Autodesk Inventor part; units mm, degrees
ref_plane "YZ Plane" through (0, 0, 0) normal (1, 0, 0) x (0, 1, 0)
ref_plane "XZ Plane" through (0, 0, 0) normal (0, 1, 0) x (-1, 0, 0)
ref_plane "XY Plane" through (0, 0, 0) normal (0, 0, 1) x (1, 0, 0)
sketch "スケッチ1" plane through (0, 0, 0) normal (0, 1, 0) x (-1, 0, 0)
  circle A0 centre (0, 0) radius 34.996
  circle A1 centre (0, 18) radius 10
  line L0 (48.9944, 0) -> (-48.9944, 0)
  line L1 (-14, 8) -> (14, 8)
  line L2 (14, 8) -> (14, 32.0737)
  line L3 (14, 32.0737) -> (-14, 32.0737)
  line L4 (-14, 32.0737) -> (-14, 8)
  line L5 (-14, 8) -> (14, 32.0737) construction
  line L6 (14, 8) -> (-14, 32.0737) construction
  point P0 (10, 25)
  point P1 (-10, 25)
  point P2 (0, 20.0368)
  dimension "d0" = 25
  dimension "d1" = 10
  dimension "d2" = 10
  dimension "d3" = 69.992
  dimension "d5" = 20
  dimension "d7" = 18
  dimension "d8" = 4
extrude "押し出し1" add sketch "スケッチ1" along normal blind 27 contours L3 A0 | A1 | L2 L1 L4 L3
hole "穴1" at (-10, 0, 25) at (10, 0, 25) direction (0, 1, 0) diameter 3.4 end through all
sketch "スケッチ2" plane through (0, 0, 0) normal (0, -1, 0) x (1, 0, 0)
  circle A0 centre (3.5, 18) radius 7 construction
  circle A1 centre (-7, 18) radius 3.5 construction
  line L0 (-3.5, 18) -> (3.5, 18) construction
  line L1 (-3.5, 11) -> (3.5, 11)
  line L2 (3.5, 25) -> (-3.5, 25)
  arc A2 (-3.5, 25) -> (-3.5, 11) centre (-3.5, 18) ccw
  arc A3 (3.5, 11) -> (3.5, 25) centre (3.5, 18) ccw
  point P0 (0, 0)
  point P1 (0, 18)
  point P2 (-10.5, 18)
  dimension "d31" = 7
  dimension "d30" = 14
  dimension "d32" = 7
extrude "押し出し2" cut sketch "スケッチ2" against normal through all
sketch "スケッチ3" plane through (0, 0, 0) normal (0, -1, 0) x (1, 0, 0)
  line L0 (14, 8) -> (-14, 8)
  line L1 (14, -21) -> (-14, -21)
  line L2 (-14, -21) -> (-14, 21)
  line L3 (-14, 21) -> (14, 21)
  line L4 (14, 21) -> (14, -21)
  line L5 (14, -21) -> (-14, 21) construction
  line L6 (-14, -21) -> (14, 21) construction
  circle A0 centre (-10, 25) radius 1.7
  point P0 (0, 0)
  point P1 (-14, 8)
  dimension "d25" = 4
extrude "押し出し3" cut sketch "スケッチ3" against normal blind 15 contours L0 L2 L3 L4
fillet "フィレット2" radius 2 8 edges at (14, 21, 8) (14, 7.5, 21) (-14, 7.5, 21) (-14, 21, 8) (14, 13.5, 32.0737) (-14, 13.5, 32.0737) (9.8246, 7.5, 21) (-9.8246, 7.5, 21)
equation "\"d32\" = 0.5 * d30"
properties part number "scara-base13" material "ABS プラスチック"
Design review of the part built by this model. Coordinates are the model's own, in mm. A direction names the side the tool comes from. Give positions to 0.01 mm unless a question says otherwise; leave off trailing zeros. Write each loop counter-clockwise with the first axis right and the second up, starting at its lowest first coordinate (ties: lowest second). Pieces come first, ordered by that corner, then holes. Notation, with made-up numbers: (85, 1.25) - (93, 1.25) arc R17 cw to (93, 23.25) - close; hole circle Ø10 at (-6.75, -14.75). An arc over 180 degrees is marked (long way). Return JSON: item names as keys, results as strings. Group by question number.
(1) We need section B-B, the plane y = 2.5. Give the boundary of the cut face in (x, z), then the cut area to 3 significant figures.
(2) We need section C-C, the plane z = 23.75. Give the boundary of the cut face in (x, y).
(3) We need section D-D, the plane y = 17.5. Give the boundary of the cut face in (x, z), then the cut area to 3 significant figures.
(4) To check wall thickness, follow probe 1 along X at (y, z) = (11, 26); probe 2 along Z at (x, y) = (-1, 22.5); probe 3 along Z at (x, y) = (10, 13.5). State the ranges of each line that lie inside material, in increasing order.
(5) Mouldability with a two-part tool opening along X and no side actions: class faces 1 (the flat face through (0, 21, 8)), 2 (the cylindrical face through (13.43, 21.08, 8.6)), 3 (the cylindrical face through (0.182, 13.311, 34.996)), 4 (the flat face through (0, 13, 25)) as +X half, -X half, draft (parallel to the pull), parting line (faces both ways), or undercut.
(6) We need section A-A, the plane x = -10. Give the boundary of the cut face in (y, z).
(7) Insertion check: pin 1 (6 mm diameter, centred on x = 6.5, z = 20.5, fed in from +Y); pin 2 (2 mm diameter, centred on x = 3, y = 11, fed in from -Z); pin 3 (5.5 mm diameter, centred on x = 1.5, y = 21.5, fed in from +Z); pin 4 (1.1 mm diameter, centred on x = -11.5, y = 4, fed in from -Z). Each pin has a flat end and moves straight along its axis. Give the tip position at first contact, or say it passes through.
(8) Machinability: for faces 5 (the cylindrical face through (-13.4, 7.6, 21.57)), 6 (the cylindrical face through (10.03, 7.4, 21.24)), 7 (the cylindrical face through (10.13, 16.31, 20.25)), 8 (the cylindrical face through (13.43, 7.6, 21.6)), 9 (the flat face through (-11.5, 7.4, 21)), which of the approach directions +Z, -Z, +X, -X, +Y, -Y give a long, thin tool a straight path to every point of the face, cutting with its end or side? Answer none if there is none.
Reported:
{
 "1": {"outline": "(-14, 23) arc R2 ccw to (-12, 21) - (-10.98, 21) arc R2 ccw to (-9.32, 21.89) arc R7 cw to (-3.5, 25) - (3.5, 25) arc R7 cw to (9.32, 21.89) arc R2 ccw to (10.98, 21) - (12, 21) arc R2 ccw to (14, 23) - (14, 30.74) arc R2 ccw to (12.73, 32.6) arc R35 ccw to (-12.73, 32.6) arc R2 ccw to (-14, 30.74) - close; hole circle Ø3.4 at (-10, 25); hole circle Ø3.4 at (10, 25)", "area": "280 mm2"},
 "2": {"outline": "(-14, 0) - (-11.15, 0) - (-11.15, 27) - (-14, 27) - close; (-8.85, 0) - (-7.49, 0) - (-7.49, 27) - (-8.85, 27) - close; (7.49, 0) - (8.85, 0) - (8.85, 27) - (7.49, 27) - close; (11.15, 0) - (14, 0) - (14, 27) - (11.15, 27) - close"},
 "3": {"outline": "(-14, 10) arc R2 ccw to (-12, 8) - (12, 8) arc R2 ccw to (14, 10) - (14, 30.74) arc R2 ccw to (12.73, 32.6) arc R35 ccw to (-12.73, 32.6) arc R2 ccw to (-14, 30.74) - close; hole circle Ø3.4 at (-10, 25); hole (-3.5, 11) - (3.5, 11) arc R7 ccw to (3.5, 25) - (-3.5, 25) arc R7 ccw to start; hole circle Ø3.4 at (10, 25)", "area": "457 mm2"},
 "4": {"probe 1": "x = -14 to -11.37, -8.63 to 8.63, 11.37 to 14", "probe 2": "z = 8 to 11, 25 to 34.98", "probe 3": "z = 21.26 to 23.3, 26.7 to 33.54"},
 "5": {"face 1": "draft", "face 2": "+X half", "face 3": "parting line", "face 4": "undercut"},
 "6": {"outline": "(0, 21.26) - (15, 21.26) - (15, 20.6) - (27, 20.6) - (27, 23.3) - (0, 23.3) - close; (0, 26.7) - (27, 26.7) - (27, 33.54) - (0, 33.54) - close; (15, 8) - (27, 8) - (27, 15.4) - (15, 15.4) - close"},
 "7": {"pin 1": "passes through", "pin 2": "stops at z = 24.98", "pin 3": "stops at z = 35", "pin 4": "stops at z = 21"},
 "8": {"face 5": "-Z, -X, -Y", "face 6": "-Z, -Y", "face 7": "+Y, -Y", "face 8": "-Z, +X, -Y", "face 9": "-Z, +X, -X, -Y"}
}
